Read the model definition and answer for the solid it produces. Units are mm, in the model's axes. A direction names the side the tool comes from. Round coordinates to 2 decimals unless told otherwise and drop trailing zeros. Write each loop counter-clockwise with the first axis right and the second up, starting at its lowest first coordinate (ties: lowest second). Pieces come first, ordered by that corner, then holes.
from build123d import *

# Parameters (mm, degrees)
BOSS_EXTRUDE2_DEPTH       = 96
CUT_EXTRUDE1_REACH        = 7
CHAMFER1_SIZE             = 2.5
F_4_0MM_DOWEL_HOLE1_D     = 4
F_4_0MM_DOWEL_HOLE1_DEPTH = 4
M4X0_7_TAPPED_HOLE1_D     = 3.3
M4X0_7_TAPPED_HOLE1_DEPTH = 4
M4X0_7_TAPPED_HOLE1_TIP   = 0.991420021


with BuildPart() as part:
    # Sketch3 → Boss-Extrude2 (new body)
    with BuildSketch(Plane(origin=(0, 0, 0), x_dir=(0, 0, -1), z_dir=(1, 0, 0))):
        Polygon((-20, 5), (-17.5, 0), (17.5, 0), (20, 5), align=None)
    extrude(amount=BOSS_EXTRUDE2_DEPTH)

    # Sketch5 → Cut-Extrude1 (cut, up to next)
    with BuildSketch(Plane(origin=(0, 5, 0), x_dir=(1, 0, 0), z_dir=(0, 1, 0)), mode=Mode.PRIVATE) as cut_extrude1_sk1:
        Polygon((0, 15), (12.5, 20), (0, 20), align=None)
    cut_extrude1_tool1 = extrude(cut_extrude1_sk1.sketch, amount=-CUT_EXTRUDE1_REACH, mode=Mode.PRIVATE) & part.part
    add(cut_extrude1_tool1.solids().sort_by_distance((4.166667, 5, -18.333333))[0], mode=Mode.SUBTRACT)
    # Sketch5 → Cut-Extrude1 (cut, up to next)
    with BuildSketch(Plane(origin=(0, 5, 0), x_dir=(1, 0, 0), z_dir=(0, 1, 0)), mode=Mode.PRIVATE) as cut_extrude1_sk2:
        Polygon((0, -20), (0, -15), (12.5, -20), align=None)
    cut_extrude1_tool2 = extrude(cut_extrude1_sk2.sketch, amount=-CUT_EXTRUDE1_REACH, mode=Mode.PRIVATE) & part.part
    add(cut_extrude1_tool2.solids().sort_by_distance((4.166667, 5, 18.333333))[0], mode=Mode.SUBTRACT)

    # Chamfer1
    chamfer1_edges = [part.edges().sort_by_distance(p)[0] for p in [
        (6.25, 5, -17.5),
        (6.25, 5, 17.5),
    ]]
    chamfer(chamfer1_edges, length=CHAMFER1_SIZE)

    # Ø4.0mm Dowel Hole1
    with Locations(Plane(origin=(0, 0, 0), x_dir=(-1, 0, 0), z_dir=(0, -1, 0))):
        with Locations((-23, 9), (-80, -9)):
            Hole(F_4_0MM_DOWEL_HOLE1_D / 2, depth=F_4_0MM_DOWEL_HOLE1_DEPTH)

    # M4x0.7 Tapped Hole1
    with Locations(Plane(origin=(0, 0, 0), x_dir=(-1, 0, 0), z_dir=(0, -1, 0))):
        with Locations((-23, -9), (-80, 9)):
            Hole(M4X0_7_TAPPED_HOLE1_D / 2, depth=M4X0_7_TAPPED_HOLE1_DEPTH)
            with Locations((0, 0, -(M4X0_7_TAPPED_HOLE1_DEPTH + M4X0_7_TAPPED_HOLE1_TIP / 2))):  # 118° drill point
                Cone(0, M4X0_7_TAPPED_HOLE1_D / 2, M4X0_7_TAPPED_HOLE1_TIP, mode=Mode.SUBTRACT)


solid = part.part
Q1. Which of the six approach directions +Z, -Z, +X, -X, +Y, -Y give full straight-line access (tool end or side, diameter ignored) to faces 1 (the flat face through (23, 4, -9)), 2 (the flat face through (3.58, 1.27, -16.43))?
Verdict:
face 1: -Y
face 2: -Z, -X, +Y, -Y
Q2. Flat-ended cylindrical pins translate along their axes: pin 1 Ø1.5 at (x, y) = (72, 3) entering from +Z (3 decimals); pin 2 Ø2.5 at (x, z) = (80, 9) entering from -Y. Find the tip coordinate at first contact, or state that the pin passes through.
Verdict:
pin 1: stops at z = 19.375
pin 2: stops at y = 4
Q3. Determine the mould class of faces 3 (the conical face through (79.7, 4.8, -9.1)), 4 (the flat face through (50, 3, 19)), 5 (the flat face through (3.58, 1.27, 16.43)) for opening direction X: pulls with the +X half, pulls with the -X half, needs draft (parallel to the pull), parting line crosses it, or undercut.
Verdict:
face 3: undercut
face 4: needs draft
face 5: pulls with the -X half
Q4. Section B-B (x = 54) is taken. Determine the outline of the cut face in (y, z).
Verdict:
outline: (0, -17.5) - (5, -20) - (5, 20) - (0, 17.5) - close
Q5. Straight lines are drawn through the part: probe 1 along Z at (x, y) = (80, 2.5); probe 2 along X at (y, z) = (1.65, 9); probe 3 along X at (y, z) = (3.05, -9.5). For each, find the intervals that lie inside material, in ascending order.
Verdict:
probe 1: z = -18.75 to -10.65, -7.35 to 7, 11 to 18.75
probe 2: x = 0 to 21.35, 24.65 to 78, 82 to 96
probe 3: x = 0 to 21.06, 24.94 to 78.43, 81.57 to 96
Q6. Section A-A (y = 1.1) is taken. Determine the outline of the cut face in (x, z) (3 decimals).
Verdict:
outline: (0, -15) - (7.625, -18.05) - (96, -18.05) - (96, 18.05) - (7.625, 18.05) - (0, 15) - close; hole circle Ø4 at (23, -9); hole circle Ø3.3 at (23, 9); hole circle Ø4 at (80, 9); hole circle Ø3.3 at (80, -9)
Q7. Section C-C (x = 17.5) is taken. Determine the outline of the cut face in (y, z), then the cut area to 3 significant figures.
Verdict:
outline: (0, -17.5) - (4.56, -19.78) - (5, -19.31) - (5, 19.31) - (4.56, 19.78) - (0, 17.5) - close
area: 187 mm2
